```python
from build123d import *

# Parameters (mm, degrees)
F1_DEPTH = 16
F2_D     = 8
F4_D     = 4


with BuildPart() as f1:
    # F0 (on Front) → F1 (new body)
    with BuildSketch(Plane.XZ):
        with BuildLine():
            Line((-8, 2.5), (-20, 2.5))
            Line((-20, 2.5), (-20, -2.5))
            Line((-20, -2.5), (20, -2.5))
            Line((20, -2.5), (20, 2.5))
            Line((20, 2.5), (8, 2.5))
            Line((8, 2.5), (8, 28.5))
            ThreePointArc((8, 28.5), (0, 36.5), (-8, 28.5))
            Line((-8, 28.5), (-8, 2.5))
        make_face()
    extrude(amount=F1_DEPTH)

    # F2 (through all)
    with Locations(Plane(origin=(0, 0, 0), x_dir=(1, 0, 0), z_dir=(0, 1, 0))):
        with Locations((0, -28.5)):
            Hole(F2_D / 2)

    # F4 (through all)
    with Locations(Plane(origin=(0, 0, -2.5), x_dir=(1, 0, 0), z_dir=(0, 0, -1))):
        with Locations((-14, 8), (14, 8)):
            Hole(F4_D / 2)


solid = f1.part
```
Can you work these out from the model? Positions are in its coordinate system, mm. A direction names the side the tool comes from. Coordinates: 2 decimals unless noted, no trailing zeros. Write each loop counter-clockwise with the first axis right and the second up, starting at its lowest first coordinate (ties: lowest second). Pieces come first, ordered by that corner, then holes. Notation, with made-up numbers: M 77.5,50 L 134.5,50 A32 cw 134.5,86 Z; hole C 42,-31 d5. An arc over 180 degrees is marked long. Write item = value, one per line. Start each with the question number.
Q1. I'm going to push flat-ended pins straight in: pin 1 (5 mm diameter, centred on y = -11.5, z = 14.5, fed in from +X); pin 2 (6.5 mm diameter, centred on x = -14, y = -8, fed in from +Z). Where does each tip first touch, or does it pass through?
Q2. If we section it at C-C, the plane y = -11: Write out the boundary of the cut face in (x, z).
Q3. If we section it at B-B, the plane x = 0: Write out the boundary of the cut face in (y, z).
Q4. On a 3-axis mill with a long thin cutter (end or side, diameter ignored), from which of +Z, -Z, +X, -X, +Y, -Y can I reach the whole of each face in a straight line? I mean faces 4 (the face through (-8, -8, 16)), 5 (the face through (13, -6, 2.5)), 6 (the face through (-20, -8, 0)). Say none if no direction works.
Q5. Thinking about a two-plate mould opening in X: for faces 1 (the face through (14, -10, 0)), 2 (the face through (-15, -6, 2.5)), 3 (the face through (8, -8, 15)), which applies, released by +X, released by -X, zero draft, split by the parting line, or undercut?
Q6. If we section it at D-D, the plane z = 31.5: Write out the boundary of the cut face in (x, y).
Q7. If I drill on L1, parallel to Z at x = 0, y = -12; L2, parallel to Y at x = 14, z = -0.9; L3, parallel to Z at x = 12.5, y = -6, over which ranges is the centre line in solid material (lowest first)? Write a range as [from, to].
Q8. If we section it at A-A, the plane y = -8.5: Write out the boundary of the cut face in (x, z).
Check sheet entries:
q1.pin_1 = 8
q1.pin_2 = 2.5
q2.outline = M -20,-2.5 L 20,-2.5 L 20,2.5 L 8,2.5 L 8,28.5 A8 ccw -8,28.5 L -8,2.5 L -20,2.5 Z; hole C 0,28.5 d8
q3.outline = M -16,-2.5 L 0,-2.5 L 0,24.5 L -16,24.5 Z; M -16,32.5 L 0,32.5 L 0,36.5 L -16,36.5 Z
q4.face_4 = +Z, -X, +Y, -Y
q4.face_5 = +Z, +X, +Y, -Y
q4.face_6 = +Z, -Z, -X, +Y, -Y
q5.face_1 = undercut
q5.face_2 = zero draft
q5.face_3 = released by +X
q6.outline = M -7.42,-16 L -2.65,-16 L -2.65,0 L -7.42,0 Z; M 2.65,-16 L 7.42,-16 L 7.42,0 L 2.65,0 Z
q7.L1 = [-2.5, 24.5], [32.5, 36.5]
q7.L2 = [-16, -10], [-6, 0]
q7.L3 = [-2.5, 2.5]
q8.outline = M -20,-2.5 L -15.94,-2.5 L -15.94,2.5 L -20,2.5 Z; M -12.06,-2.5 L 12.06,-2.5 L 12.06,2.5 L 8,2.5 L 8,28.5 A8 ccw -8,28.5 L -8,2.5 L -12.06,2.5 Z; M 15.94,-2.5 L 20,-2.5 L 20,2.5 L 15.94,2.5 Z; hole C 0,28.5 d8
